Solid Edge part; units mm, degrees
sketch "Sketch1" plane through (0, 0, 0) normal (0, 0, 1) x (1, 0, 0)
  line L0 (0, 0) -> (124.5, 0)
  line L1 (124.5, 0) -> (124.5, 54)
  line L2 (124.5, 54) -> (0, 54)
  line L3 (0, 54) -> (0, 0)
extrude "Protrusion1" add sketch "Sketch1" along normal up to vertex (15 mm away) and the other way up to vertex (17.5 mm away)
chamfer "Chamfer1" distance 5 angle 45 4 edges at (0, 0, -1.25) (124.5, 0, -1.25) (124.5, 54, -1.25) (0, 54, -1.25)
sketch "Sketch2" plane through (62.25, 27, 15) normal (0, 0, 1) x (1, 0, 0)
  line L0 (-56.25, 11.6) -> (-40.25, 11.6)
  arc A0 (-40.25, 11.6) -> (-36.75, 15.1) centre (-40.25, 15.1) ccw
  arc A1 (-36.75, 15.1) -> (-40.25, 18.6) centre (-40.25, 15.1) ccw
  line L1 (-40.25, 18.6) -> (-56.25, 18.6)
  arc A2 (-56.25, 18.6) -> (-58.9973, 12.9315) centre (-56.25, 15.1) ccw
  arc A3 (-56.25, 11.6) -> (-58.9973, 12.9315) centre (-56.25, 15.1) cw
extrude "Cutout1" cut sketch "Sketch2" against normal through all
pattern_linear "Pattern1" count 2 spacing 96.5 along (1, 0, 0) count 2 spacing 30.2 along (0, -1, 0) of "Cutout1"
sketch "Sketch3" plane through (62.25, 27, 15) normal (0, 0, 1) x (1, 0, 0)
  line L0 (32.5, 14.5) -> (-32.5, 14.5)
  line L1 (-32.5, 14.5) -> (-32.5, -14.5)
  line L2 (-32.5, -14.5) -> (32.5, -14.5)
  line L3 (32.5, -14.5) -> (32.5, 14.5)
extrude "Cutout2" cut sketch "Sketch3" against normal through all
sketch "Sketch4" plane through (62.25, 27, 15) normal (0, 0, 1) x (1, 0, 0)
  line L0 (32.5, 23) -> (-32.5, 23)
  line L1 (-32.5, 23) -> (-32.5, -23)
  line L2 (-32.5, -23) -> (32.5, -23)
  line L3 (32.5, -23) -> (32.5, 23)
extrude "VaciadoExtruido_3" cut sketch "Sketch4" against normal blind 13
fillet "Redondeo_1" radius 5 8 edges at (29.75, 50, 8.5) (94.75, 50, 8.5) (94.75, 4, 8.5) (94.75, 12.5, -7.75) (94.75, 41.5, -7.75) (29.75, 41.5, -7.75) (29.75, 4, 8.5) (29.75, 12.5, -7.75)
sketch "Sketch5" plane through (62.25, 27, -17.5) normal (0, 0, -1) x (-1, 0, 0)
  line L0 (-32.5, 23) -> (-32.5, -23)
  line L1 (-32.5, -23) -> (32.5, -23)
  line L2 (32.5, -23) -> (32.5, 23)
  line L3 (32.5, 23) -> (-32.5, 23)
extrude "Protrusion2" add sketch "Sketch5" against normal up to vertex (14 mm away)
sketch "Sketch6" plane through (62.25, 27, -17.5) normal (0, 0, -1) x (-1, 0, 0)
  circle A0 centre (16.5, 0) radius 8.5
extrude "Cutout3" cut sketch "Sketch6" against normal up to vertex (14 mm away)
hole "Agujero_1" at (41.75, 9.7, 2) direction (0, 0, -1) diameter 3 end through all
hole "Hole1" at (63.75, 9.7, 2) direction (0, 0, -1) diameter 3 end through all
hole "Hole2" at (85.75, 9.7, 2) direction (0, 0, -1) diameter 3 end through all
hole "Hole3" at (41.75, 44.3, 2) direction (0, 0, -1) diameter 3 end through all
hole "Hole4" at (63.75, 44.3, 2) direction (0, 0, -1) diameter 3 end through all
hole "Hole5" at (85.75, 44.3, 2) direction (0, 0, -1) diameter 3 end through all
sketch "Sketch7" plane through (14, 27, -14) normal (0, 0, -1) x (-1, 0, 0)
  line L0 (15.0837, -36.0096) -> (-114.5837, -36.0096)
  line L1 (-114.5837, -36.0096) -> (-114.5837, 36.0096)
  line L2 (-114.5837, 36.0096) -> (15.0837, 36.0096)
  line L3 (15.0837, 36.0096) -> (15.0837, -36.0096)
extrude "VaciadoExtruido_8" cut sketch "Sketch7" along normal through all
hole "Agujero_7" at (41.75, 9.7, -14) direction (0, 0, 1) diameter 3 end up to next counterbore diameter 5 counterbore depth 12
hole "Hole6" at (63.75, 9.7, -14) direction (0, 0, 1) diameter 3 end up to next counterbore diameter 5 counterbore depth 12
hole "Hole7" at (85.75, 9.7, -14) direction (0, 0, 1) diameter 3 end up to next counterbore diameter 5 counterbore depth 12
hole "Hole8" at (41.75, 44.3, -14) direction (0, 0, 1) diameter 3 end up to next counterbore diameter 5 counterbore depth 12
hole "Hole9" at (63.75, 44.3, -14) direction (0, 0, 1) diameter 3 end up to next counterbore diameter 5 counterbore depth 12
hole "Hole10" at (85.75, 44.3, -14) direction (0, 0, 1) diameter 3 end up to next counterbore diameter 5 counterbore depth 12
sketch "Sketch8" plane through (62.25, 27, -3.5) normal (0, 0, 1) x (0, -1, 0)
  circle A0 centre (0, -16.5) radius 11.5
extrude "VaciadoExtruido_9" cut sketch "Sketch8" against normal blind 1
properties part number "BRAZO2" material "Aluminio, 7075-T6"
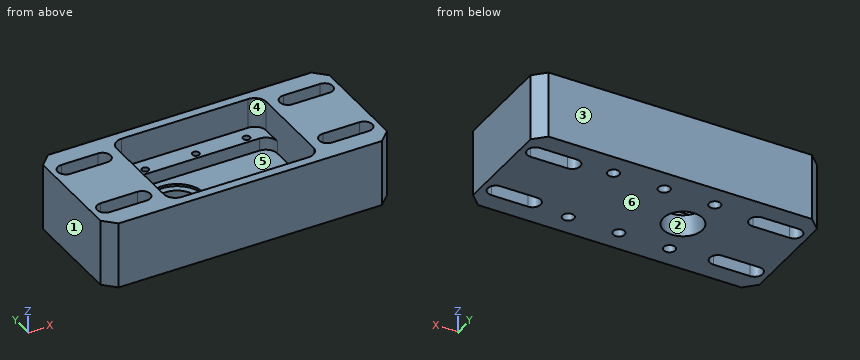
Source: CAD feature listing. Evaluate the final solid. Frame: model axes, mm. Face numbers are marked on the shaded views. A direction names the side the tool comes from. Round coordinates to 2 decimals unless told otherwise and drop trailing zeros. Loops run counter-clockwise (first coordinate to the right, second up) from the corner with the lowest first, then second, coordinate; pieces in that order, holes last. Notation, with made-up numbers: (81.5, 30.25) - (129.5, 30.25) arc R33 ccw to (129.5, 60.25) - close; hole circle Ø7 at (65.25, 56.25). An arc over 180 degrees is marked (long way). Write item = value, one per line. Start each with the question number.
Item 1: First-contact query: pin 1 Ø14 at (x, y) = (45.75, 27) entering from +Z; pin 2 Ø4 at (x, y) = (85.75, 44.3) entering from +Z. Flat tips, straight axial feed; report the tip coordinate or a pass-through.
Item 2: Material intervals for line 1 (Y direction, x = 110.5, z = 6.5); line 2 (Y direction, x = 64, z = -7); line 3 (Y direction, x = 63.75, z = 1), sorted ascending.
Item 3: Section query B-B on z = 13. Count the separate pieces of the cut face and the enclosed holes in it, plus the area to 3 significant figures.
Item 4: Mould query, pull axis X, two halves, no side actions, for the marked faces 1, 2, 3 and 4. Classes: released by +X, released by -X, zero draft, split by the parting line, or undercut.
Item 5: Section query C-C on x = 45.75. Output: boundary loops of the cut face in (y, z).
Item 6: Reachability of the marked faces 5 and 6 from +Z, -Z, +X, -X, +Y, -Y: full face, straight path, thin tool, end or side. Return the list, or none.
Item 7: Section query A-A on x = 63.75. Output: boundary loops of the cut face in (y, z), plus the area to 4 significant figures.
Item 8: Section query D-D on x = 108. Output: boundary loops of the cut face in (y, z), plus the area to 3 significant figures.
Results list:
q1.pin_1 = through
q1.pin_2 = 2
q2.line_1 = 0 to 8.4, 15.4 to 38.6, 45.6 to 54
q2.line_2 = 0 to 7.21, 12.19 to 41.81, 46.79 to 54
q2.line_3 = 0 to 8.2, 11.2 to 12.5, 41.5 to 42.8, 45.8 to 54
q3.separate_pieces = 1
q3.enclosed_holes = 5
q3.area = 3,100 mm²
q4.face_1 = released by -X
q4.face_2 = undercut
q4.face_3 = zero draft
q4.face_4 = undercut
q5.outline = (0, -14) - (18.5, -14) - (18.5, -4.5) - (15.5, -4.5) - (15.5, -3.5) - (12.5, -3.5) - (12.5, 2) - (4, 2) - (4, 15) - (0, 15) - close; (35.5, -14) - (54, -14) - (54, 15) - (50, 15) - (50, 2) - (41.5, 2) - (41.5, -3.5) - (38.5, -3.5) - (38.5, -4.5) - (35.5, -4.5) - close
q6.face_5 = +Z
q6.face_6 = -Z, +X, -X, +Y, -Y
q7.outline = (0, -14) - (7.2, -14) - (7.2, -2) - (8.2, -2) - (8.2, 2) - (4, 2) - (4, 15) - (0, 15) - close; (11.2, -2) - (12.2, -2) - (12.2, -14) - (41.8, -14) - (41.8, -2) - (42.8, -2) - (42.8, 2) - (41.5, 2) - (41.5, -3.5) - (12.5, -3.5) - (12.5, 2) - (11.2, 2) - close; (45.8, -2) - (46.8, -2) - (46.8, -14) - (54, -14) - (54, 15) - (50, 15) - (50, 2) - (45.8, 2) - close
q7.area = 664.5 mm²
q8.outline = (0, -14) - (8.4, -14) - (8.4, 15) - (0, 15) - close; (15.4, -14) - (38.6, -14) - (38.6, 15) - (15.4, 15) - close; (45.6, -14) - (54, -14) - (54, 15) - (45.6, 15) - close
q8.area = 1,160 mm²
